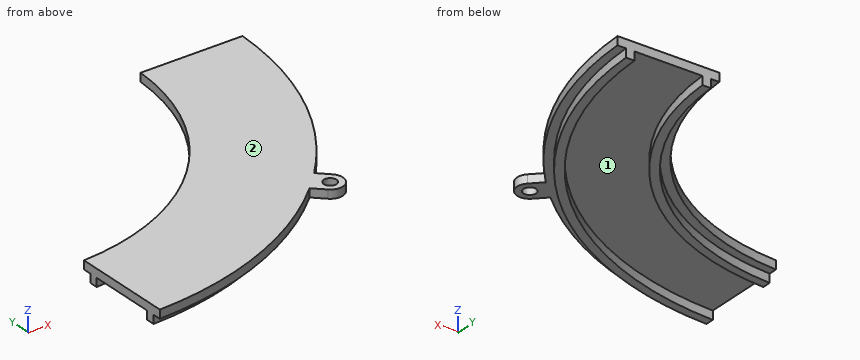
```python
from build123d import *

# Parameters (mm, degrees)
EXTRUDE_1_DEPTH = 2
EXTRUDE_2_DEPTH = 2
EXTRUDE_START   = -2
SKETCH_4_R      = 1.5
EXTRUDE_3_DEPTH = 2


with BuildPart() as part:
    # 草图2 → 凸台-拉伸1 (new body)
    with BuildSketch(Plane.XY):
        with BuildLine():
            Line((3, -77.441913716), (3, -79.443376061))
            ThreePointArc((3, -79.443376061), (56.214989104, -56.214989104), (79.443376061, -3))
            Line((79.443376061, -3), (77.441913716, -3))
            Line((77.441913716, -3), (55.418859606, -3))
            ThreePointArc((55.418859606, -3), (39.244426356, -39.244426356), (3, -55.418859606))
            Line((3, -55.418859606), (3, -77.441913716))
        make_face()
    extrude(amount=EXTRUDE_1_DEPTH)

    # 草图3 → 凸台-拉伸2 (add)
    with BuildSketch(Plane.XY):
        with BuildLine():
            Line((3, -57.421685799), (3, -59.42432162))
            ThreePointArc((3, -59.42432162), (42.072853481, -42.072853481), (59.42432162, -3))
            Line((59.42432162, -3), (57.421685799, -3))
            ThreePointArc((57.421685799, -3), (40.658639918, -40.658639918), (3, -57.421685799))
        make_face()
        with BuildLine():
            Line((77.441913716, -3), (75.440373806, -3))
            ThreePointArc((75.440373806, -3), (53.38656198, -53.38656198), (3, -75.440373806))
            Line((3, -75.440373806), (3, -77.441913716))
            ThreePointArc((3, -77.441913716), (54.800775542, -54.800775542), (77.441913716, -3))
        make_face()
    extrude(amount=-EXTRUDE_2_DEPTH)

    # 草图4 → 凸台-拉伸3 (add)
    with BuildSketch(Plane.XY.offset(2).offset(EXTRUDE_START)):
        with BuildLine():
            ThreePointArc((58.296270277, -54.05362959), (56.214989104, -56.214989104), (54.05362959, -58.296270277))
            Line((54.05362959, -58.296270277), (56.528503324, -60.771144011))
            ThreePointArc((56.528503324, -60.771144011), (60.771144011, -60.771144011), (60.771144011, -56.528503324))
            Line((60.771144011, -56.528503324), (58.296270277, -54.05362959))
        make_face()
        with Locations((58.649823667, -58.649823667)):
            Circle(SKETCH_4_R, mode=Mode.SUBTRACT)
    extrude(amount=EXTRUDE_3_DEPTH)


solid = part.part
```
Design review of the part built by this model. Coordinates are the model's own, in mm. Face numbers are marked on the shaded views. Give positions to 0.01 mm unless a question says otherwise; leave off trailing zeros. Order: outer loops, then holes, each group sorted by start corner. A loop starts at its lowest first (then second) coordinate and runs counter-clockwise, first axis right, second up. Notation, with made-up numbers: (44.25, 0) -> (95.25, 0) arc R20 cw to (95.25, 24) -> close; hole circle Ø5 at (-29, 75). An arc over 180 degrees is marked (long way). Write each question's results on one line, items separated by ' | '. Start each with the question number.
Q1. Wall thickness on L1, parallel to Z at x = 76.5, y = -13.5; L2, parallel to X at y = -38.5, z = -0.7; L3, parallel to Y at x = 24.5, z = -1.05: over which ranges is each line inside the solid? List them lowest first. Write a range as from..to.
Q2. Add section A-A on z = -0.65. Give the boundary of the cut face in (x, y).
Q3. For pin 1 (1.8 mm diameter, centred on x = 58.65, y = -58.65, fed in from -Z); pin 2 (2 mm diameter, centred on y = -42, z = 1, fed in from +X); pin 3 (1.5 mm diameter, centred on y = -27, z = -1, fed in from -X); pin 4 (1.5 mm diameter, centred on y = -60, z = 1, fed in from +X), all flat-tipped, find the tip position at first contact; note any pin that passes through.
Q4. Add section C-C on y = -74. Give the boundary of the cut face in (x, z), and give its area (3 significant figures).
Q5. Add section D-D on x = 32.5. Give the boundary of the cut face in (y, z).
Q6. Mouldability with a two-part tool opening along Y and no side actions: class the marked faces 1 and 2 as +Y half, -Y half, draft (parallel to the pull), parting line (faces both ways), or undercut.
Q7. Add section B-B on x = 47. Give the boundary of the cut face in (y, z), and give its area (3 significant figures).
Found:
1) L1: z = 0..2 | L2: x = 42.71..45.37, 64.95..67.26 | L3: y = -73.53..-71.41, -54.22..-52.02
2) outline: (3, -77.44) arc R77.5 ccw to (77.44, -3) -> (75.44, -3) arc R75.5 cw to (3, -75.44) -> close; (3, -59.42) arc R59.5 ccw to (59.42, -3) -> (57.42, -3) arc R57.5 cw to (3, -57.42) -> close
3) pin 1: passes through | pin 2: stops at x = 68.11 | pin 3: stops at x = 50.36 | pin 4: stops at x = 61.59
4) outline: (3, 0) -> (14.97, 0) -> (14.97, -2) -> (23.03, -2) -> (23.03, 0) -> (29.06, 0) -> (29.06, 2) -> (3, 2) -> close | area: 68.2 mm2
5) outline: (-72.55, 0) -> (-70.36, 0) -> (-70.36, -2) -> (-68.15, -2) -> (-68.15, 0) -> (-49.84, 0) -> (-49.84, -2) -> (-47.43, -2) -> (-47.43, 0) -> (-44.99, 0) -> (-44.99, 2) -> (-72.55, 2) -> close
6) face 1: undercut | face 2: draft
7) outline: (-64.12, 0) -> (-61.62, 0) -> (-61.62, -2) -> (-59.09, -2) -> (-59.09, 0) -> (-36.49, 0) -> (-36.49, -2) -> (-33.12, -2) -> (-33.12, 0) -> (-29.52, 0) -> (-29.52, 2) -> (-64.12, 2) -> close | area: 81.0 mm2
